```python
from build123d import *

# Parameters (mm, degrees)
SKETCH_1_R          = 55
EXTRUDE_1_DEPTH     = 30
SKETCH_3_R          = 49.5
CUT_EXTRUDE_1_DEPTH = 25
SKETCH_5_W          = 47
SKETCH_5_H          = 12.24289715
CUT_EXTRUDE_2_DEPTH = 30
FILLET_4_R          = 2
FILLET_5_R          = 2
SKETCH_6_R          = 6.65
CUT_EXTRUDE_3_DEPTH = 12
EXTRUDE_START       = -5
EXTRUDE_3_DEPTH     = 5
FILLET_7_R          = 10
FILLET_8_R          = 5
SKETCH_10_R         = 3
CUT_EXTRUDE_5_DEPTH = 5


with BuildPart() as part:
    # 草图1 → 凸台-拉伸1 (new body)
    with BuildSketch(Plane(origin=(0, 0, 0), x_dir=(1, 0, 0), z_dir=(0, 1, 0))):
        with Locations(Location((0, 0, 0), (0, 0, 270))):
            Circle(SKETCH_1_R)
    extrude(amount=EXTRUDE_1_DEPTH)

    # 草图3 → 切除-拉伸1 (cut)
    with BuildSketch(Plane(origin=(0, 30, 0), x_dir=(1, 0, 0), z_dir=(0, 1, 0))):
        with Locations(Location((0, 0, 0), (0, 0, 270))):
            Circle(SKETCH_3_R)
    extrude(amount=-CUT_EXTRUDE_1_DEPTH, mode=Mode.SUBTRACT)

    # 草图5 → 切除-拉伸2 (cut)
    with BuildSketch(Plane(origin=(0, 30, 0), x_dir=(1, 0, 0), z_dir=(0, 1, 0))):
        with Locations((0, 49.687490397)):
            Rectangle(SKETCH_5_W, SKETCH_5_H)
    extrude(amount=-CUT_EXTRUDE_2_DEPTH, mode=Mode.SUBTRACT)

    # 圆角4
    fillet_4_edges = [part.edges().sort_by_distance(p)[0] for p in [
        (-23.5, 15, -49.726753363),
    ]]
    fillet(fillet_4_edges, radius=FILLET_4_R)

    # 圆角5
    fillet_5_edges = [part.edges().sort_by_distance(p)[0] for p in [
        (23.5, 15, -49.726753363),
    ]]
    fillet(fillet_5_edges, radius=FILLET_5_R)

    # 草图6 → 切除-拉伸3 (cut)
    with BuildSketch(Plane(origin=(0, 5, 0), x_dir=(1, 0, 0), z_dir=(0, 1, 0))):
        with Locations(Location((0, 0, 0), (0, 0, 270))):
            Circle(SKETCH_6_R)
    extrude(amount=-CUT_EXTRUDE_3_DEPTH, mode=Mode.SUBTRACT)

    # 草图14 → 凸台-拉伸3 (add)
    with BuildSketch(Plane(origin=(0, 5, 0), x_dir=(1, 0, 0), z_dir=(0, 1, 0)).offset(EXTRUDE_START)):
        with BuildLine():
            Line((-49.898576095, 23.132922507), (-63.862525635, 37.044772973))
            Line((-63.862525635, 37.044772973), (-49.746845912, 51.213315099))
            Line((-49.746845912, 51.213315099), (-38.128637352, 39.638453724))
            ThreePointArc((-38.128637352, 39.638453724), (-44.78063998, 31.932652301), (-49.898576095, 23.132922507))
        make_face()
        with BuildLine():
            Line((49.811900188, -23.3189751), (64.421720913, -37.928795825))
            Line((64.421720913, -37.928795825), (50.279585289, -52.070931449))
            Line((50.279585289, -52.070931449), (37.984884655, -39.776230814))
            ThreePointArc((37.984884655, -39.776230814), (44.662950793, -32.097053236), (49.811900188, -23.3189751))
        make_face()
        with BuildLine():
            Line((-49.632393674, -23.698639164), (-63.862550335, -37.928795825))
            Line((-63.862550335, -37.928795825), (-49.720414711, -52.070931449))
            Line((-49.720414711, -52.070931449), (-37.697852746, -40.048369484))
            ThreePointArc((-37.697852746, -40.048369484), (-44.423770724, -32.427281642), (-49.632393674, -23.698639164))
        make_face()
        with BuildLine():
            Line((38.475737251, 39.301623923), (50.118901666, 51.212426922))
            Line((50.118901666, 51.212426922), (64.420808036, 37.231887798))
            Line((64.420808036, 37.231887798), (50.134465219, 22.6171483))
            ThreePointArc((50.134465219, 22.6171483), (45.083643676, 31.50341367), (38.475737251, 39.301623923))
        make_face()
    extrude(amount=EXTRUDE_3_DEPTH)

    # 圆角7
    fillet_7_edges = [part.edges().sort_by_distance(p)[0] for p in [
        (-38.128637352, 2.5, -39.638453724),
        (-49.898576095, 2.5, -23.132922507),
        (-49.632393674, 2.5, 23.698639164),
        (-37.697852746, 2.5, 40.048369484),
        (50.134465219, 2.5, -22.6171483),
        (38.475737251, 2.5, -39.301623923),
        (37.984884655, 2.5, 39.776230814),
        (49.811900188, 2.5, 23.3189751),
    ]]
    fillet(fillet_7_edges, radius=FILLET_7_R)

    # 圆角8
    fillet_8_edges = [part.edges().sort_by_distance(p)[0] for p in [
        (-63.862525635, 2.5, -37.044772973),
        (-49.746845912, 2.5, -51.213315099),
        (-49.720414711, 2.5, 52.070931449),
        (-63.862550335, 2.5, 37.928795825),
        (50.118901666, 2.5, -51.212426922),
        (64.420808036, 2.5, -37.231887798),
        (50.279585289, 2.5, 52.070931449),
        (64.421720913, 2.5, 37.928795825),
    ]]
    fillet(fillet_8_edges, radius=FILLET_8_R)

    # 草图10 → 切除-拉伸5 (cut)
    with BuildSketch(Plane(origin=(0, 5, 0), x_dir=(1, 0, 0), z_dir=(0, 1, 0))):
        with Locations(Location((-49.720414711, 37.071204175, 0), (0, 0, 270))):
            Circle(SKETCH_10_R)
        with Locations(Location((50.279585289, 37.071204175, 0), (0, 0, 270))):
            Circle(SKETCH_10_R)
        with Locations(Location((-49.720414711, -37.928795825, 0), (0, 0, 270))):
            Circle(SKETCH_10_R)
        with Locations(Location((50.279585289, -37.928795825, 0), (0, 0, 270))):
            Circle(SKETCH_10_R)
    extrude(amount=-CUT_EXTRUDE_5_DEPTH, mode=Mode.SUBTRACT)


solid = part.part
```
Here's how the part is built. I have some questions about the finished solid (model axes, mm). A direction names the side the tool comes from. Coordinates: 2 decimals unless noted, no trailing zeros. Order: outer loops, then holes, each group sorted by start corner. A loop starts at its lowest first (then second) coordinate and runs counter-clockwise, first axis right, second up. Notation, with made-up numbers: (37, -17.5) - (96, -17.5) arc R17 cw to (96, 10.5) - close; hole circle Ø9 at (87, 4.25). An arc over 180 degrees is marked (long way). One line per question, with ' | ' between items.
(1) If I drill on L1, parallel to X at y = 12, z = -1.5; L2, parallel to X at y = 1.5, z = 0; L3, parallel to Z at x = -41, y = 14, over which ranges is the centre line in solid material (lowest first)?
Report:
L1: x = -54.98 to -49.48, 49.48 to 54.98 | L2: x = -55 to -6.65, 6.65 to 55 | L3: z = -36.66 to -27.74, 27.74 to 36.66
(2) If we mould it in two halves opening along X, with no side actions, what happens to faces 5 (the cylindrical face through (47.618, 2.535, -35.687)), 6 (the flat face through (-56.84, 2.46, 44.95)), 7 (the flat face through (52, 5, -40))? For each: pulls with the +X half, pulls with the -X half, needs draft (parallel to the pull), parting line crosses it, or undercut.
Report:
face 5: undercut | face 6: pulls with the -X half | face 7: needs draft
(3) For faces 1 (the flat face through (0, 3, -43.566)), 2 (the flat face through (-57.4, 2.465, -30.606)), 3 (the flat face through (57.635, 2.465, 31.142)), 4 (the cylindrical face through (-52.382, 2.535, -35.687)), which set-ups out of +Z, -Z, +X, -X, +Y, -Y let a thin tool reach every point of the face, with its end or its side?
Report:
face 1: -Z, +Y, -Y | face 2: -X, +Y, -Y | face 3: +X, +Y, -Y | face 4: +Y, -Y
(4) Will these pins go through, and if not, where does the flat tip stop? pin 1 (1.5 mm diameter, centred on x = -0.5, y = 2.5, fed in from -Z); pin 2 (1 mm diameter, centred on x = 27.5, z = 13, fed in from +Y); pin 3 (4 mm diameter, centred on y = 9, z = -33.5, fed in from -X); pin 4 (5 mm diameter, centred on x = 50.28, z = 37.93, fed in from +Y).
Report:
pin 1: stops at z = -43.57 | pin 2: stops at y = 5 | pin 3: stops at x = -45.09 | pin 4: passes through
(5) Suppose I cut it at D-D on z = 31. List the corners of the cut face in (x, y) for me.
Report:
outline: (-56.93, 0) - (57.49, 0) - (57.49, 5) - (45.43, 5) - (45.43, 30) - (38.59, 30) - (38.59, 5) - (-38.59, 5) - (-38.59, 30) - (-45.43, 30) - (-45.43, 5) - (-56.93, 5) - close
(6) Suppose I cut it at C-C on y = 22. List the corners of the cut face in (x, z) for me.
Report:
outline: (-26.46, -48.22) arc R2 ccw to (-23.5, -46.46) - (-23.5, -43.57) arc R49.5 cw (long way) to (23.5, -43.57) - (23.5, -46.46) arc R2 ccw to (26.46, -48.22) arc R55 ccw (long way) to start
(7) Suppose I cut it at A-A on z = 0. List the corners of the cut face in (x, y) for me, and give its area (4 significant figures).
Report:
outline: (-55, 0) - (-6.65, 0) - (-6.65, 5) - (-49.5, 5) - (-49.5, 30) - (-55, 30) - close; (6.65, 0) - (55, 0) - (55, 30) - (49.5, 30) - (49.5, 5) - (6.65, 5) - close | area: 758.5 mm2
(8) Suppose I cut it at B-B on x = 0. List the corners of the cut face in (y, z) for me, and give its area (3 significant figures).
Report:
outline: (0, -43.57) - (5, -43.57) - (5, -6.65) - (0, -6.65) - close; (0, 6.65) - (5, 6.65) - (5, 49.5) - (30, 49.5) - (30, 55) - (0, 55) - close | area: 564 mm2
